from build123d import *

# Parameters (mm, degrees)
F1_DEPTH = 12
F2_R     = 10
F2_R_2   = 4.6
F3_DEPTH = 2
F2_R_3   = 2.6
F4_DEPTH = 12.001
F5_SIZE  = 1


with BuildPart() as f1:
    # F0 (on Top) → F1 (new body)
    with BuildSketch(Plane.XY):
        Polygon((3.464102, 6), (-3.464102, 6), (-6.928203, 0), (-3.464102, -6), (3.464102, -6), (6.928203, 0), align=None)
    extrude(amount=F1_DEPTH)

    # F2 (on Top) → F3 (join)
    with BuildSketch(Plane.XY):
        Circle(F2_R)
        Circle(F2_R_2, mode=Mode.SUBTRACT)
    extrude(amount=F3_DEPTH)

    # F2 (on Top) → F4 (cut, through all)
    with BuildSketch(Plane.XY):
        Circle(F2_R_3)
    extrude(amount=F4_DEPTH, mode=Mode.SUBTRACT)

    # F5
    f5_edges = [f1.edges().sort_by_distance(p)[0] for p in [
        (-10, 0, 2),
        (0, 6, 2),
        (-5.196152, 3, 2),
        (-5.196152, -3, 2),
        (0, -6, 2),
        (5.196152, -3, 2),
        (5.196152, 3, 2),
    ]]
    chamfer(f5_edges, length=F5_SIZE)


solid = f1.part
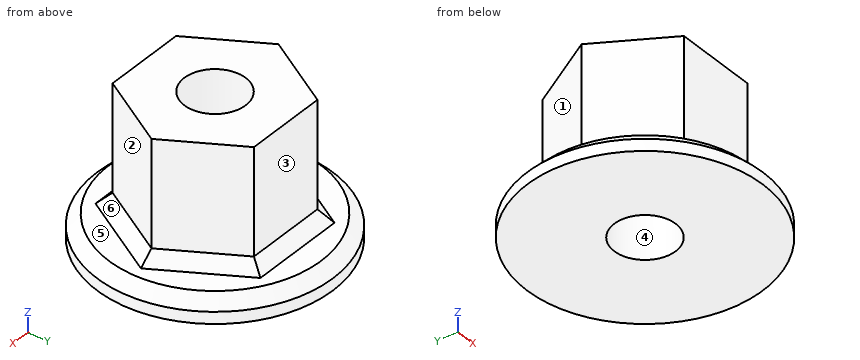
Read the model definition and answer for the solid it produces. Units are mm, in the model's axes. Face numbers are marked on the shaded views. A direction names the side the tool comes from. Coordinates: 2 decimals unless noted, no trailing zeros. Order: outer loops, then holes, each group sorted by start corner. A loop starts at its lowest first (then second) coordinate and runs counter-clockwise, first axis right, second up. Notation, with made-up numbers: M 67,71.5 L 109,71.5 A13 ccw 109,82.5 Z; hole C 59,-33 d2. An arc over 180 degrees is marked long. Put each result on its own line as item: value. Start each with the question number.
Item 1: Given pin 1 Ø4 at (y, z) = (5, 2) entering from -X; pin 2 Ø5.5 at (x, z) = (1.5, 5.5) entering from +Y; pin 3 Ø2 at (x, z) = (-1.5, 5.5) entering from -Y, each flat-ended and moving along its own axis, determine where each tip first touches the part or whether it passes through.
Item 2: The mould has two halves that part along X. Classify the marked faces 4, 5 and 6: +X half, -X half, draft (parallel to the pull), parting line (faces both ways), or undercut.
Item 3: Section A-A, the plane x = 0 is taken. Determine the outline of the cut face in (y, z).
Item 4: For the marked faces 1, 2 and 3, determine the directions among +Z, -Z, +X, -X, +Y, -Y from which every point of the face is accessible in a straight line to the end or side of a thin tool.
Item 5: Section B-B, the plane z = 9.75 is taken. Determine the outline of the cut face in (x, y).
Item 6: Section C-C, the plane z = 1.25 is taken. Determine the outline of the cut face in (x, y), plus the area to 3 significant figures.
Item 7: Consider probe 1 along Y at (x, z) = (0, 6); probe 2 along Z at (x, y) = (-7.75, 4.25); probe 3 along Y at (x, z) = (1.5, 10). Determine where each line is inside the solid, lowest interval first. Write a range as [from, to].
Computed:
1. pin 1: stops at x = -9.45
1. pin 2: stops at y = 6.25
1. pin 3: stops at y = -6
2. face 4: undercut
2. face 5: draft
2. face 6: +X half
3. outline: M -10,0 L -2.6,0 L -2.6,12 L -6,12 L -6,3 L -7,2 L -9,2 L -10,1 Z; M 2.6,0 L 10,0 L 10,1 L 9,2 L 7,2 L 6,3 L 6,12 L 2.6,12 Z
4. face 1: +Z, -X, +Y
4. face 2: +Z, +X, -Y
4. face 3: +Z, +X, -X, +Y
5. outline: M -6.93,0 L -3.46,-6 L 3.46,-6 L 6.93,0 L 3.46,6 L -3.46,6 Z; hole C 0,0 d5.2
6. outline: C 0,0 d19.5; hole C 0,0 d5.2
6. area: 277 mm2
7. probe 1: y = [-6, -2.6], [2.6, 6]
7. probe 2: z = [0, 2]
7. probe 3: y = [-6, -2.12], [2.12, 6]
